Verification items for the finished model (mm, model axes). A direction names the side the tool comes from. Coordinates: 2 decimals unless noted, no trailing zeros. Write each loop counter-clockwise with the first axis right and the second up, starting at its lowest first coordinate (ties: lowest second). Pieces come first, ordered by that corner, then holes. Notation, with made-up numbers: (34.5, 45) -> (42.5, 45) arc R17 ccw to (42.5, 73) -> close; hole circle Ø10 at (41, 35). An arc over 180 degrees is marked (long way). Answer in a Markdown table with one row per item.
Autodesk Fusion 360 part; units mm, degrees
sketch "Sketch1" plane through (0, 0, 0) normal (0, 1, 0) x (1, 0, 0)
  line L0 (2.4744, -68.9852) -> (7.4744, -68.9852)
  line L1 (7.4744, -68.9852) -> (7.4744, -22.3387)
  line L2 (7.4744, -22.3387) -> (36.754, -10.3303)
  line L3 (36.754, -10.3303) -> (34.8567, -5.7042)
  line L4 (34.8567, -5.7042) -> (2.4744, -18.9852)
  line L5 (2.4744, -18.9852) -> (2.4744, -68.9852)
  line L6 (2.4744, -68.9852) -> (7.4744, -66.9345)
  line L7 (34.8567, -5.7042) -> (34.8567, -11.1084)
  dimension "d1" = 5
  dimension "d2" = 5
  dimension "d3" = 112.3
  dimension "d16" = 50
  dimension "d18" = 22.3
  dimension "d20" = 35
extrude "Extrude1" add sketch "Sketch1" along normal blind 220 contours L1 L2 L4 L5 L6 L7
sketch "Sketch2" plane through (2.4744, 0, 0) normal (-1, 0, 0) x (0, -1, 0)
  line L0 (0, 18.9852) -> (0, 68.9852)
  line L1 (-220, 68.9852) -> (-220, 18.9852)
  line L2 (-220, 18.9852) -> (0, 18.9852)
  line L3 (-215, 66.9852) -> (-5, 66.9852)
  line L4 (-5, 66.9852) -> (-5, 56.9852)
  line L5 (-5, 56.9852) -> (-215, 56.9852)
  line L6 (-215, 56.9852) -> (-215, 66.9852)
  line L7 (-215, 52.9852) -> (-5, 52.9852)
  line L8 (-5, 52.9852) -> (-5, 42.9852)
  line L9 (-5, 42.9852) -> (-215, 42.9852)
  line L10 (-215, 42.9852) -> (-215, 52.9852)
  line L11 (-5, 66.9852) -> (-15, 66.9852)
  line L12 (-15, 56.9852) -> (-5, 56.9852)
  line L13 (-5, 56.9852) -> (-5, 66.9852)
  line L14 (-5, 52.9852) -> (-15, 52.9852)
  line L15 (-15, 42.9852) -> (-5, 42.9852)
  line L16 (-5, 42.9852) -> (-5, 52.9852)
  line L17 (0, 68.9852) -> (-220, 68.9852)
  dimension "d6" = 210
  dimension "d7" = 210
  dimension "d8" = 5
  dimension "d9" = 5
  dimension "d12" = 10
  dimension "d13" = 10
  dimension "d22" = 4
  dimension "d30" = 2
extrude "Extrude2" cut sketch "Sketch2" against normal blind 3 contours L3 L4 L5 L6 L11 L12 L13 | L7 L8 L9 L10 L14 L15 L16
sketch "Sketch3" plane through (5.4744, 0, 0) normal (-1, 0, 0) x (0, -1, 0)
  line L0 (-215, 56.9852) -> (-5, 56.9852)
  line L1 (-5, 56.9852) -> (-5, 66.9852)
  line L2 (-5, 66.9852) -> (-215, 66.9852)
  line L3 (-215, 66.9852) -> (-215, 56.9852)
  line L4 (-5, 66.9852) -> (-15, 66.9852)
  line L5 (-15, 66.9852) -> (-15, 56.9852)
  line L6 (-15, 56.9852) -> (-5, 56.9852)
  line L7 (-5, 56.9852) -> (-5, 66.9852)
  dimension "d33" = 10
  dimension "d34" = 10
sketch "Sketch4" plane through (5.4744, 0, 0) normal (-1, 0, 0) x (0, -1, 0)
  line L0 (-215, 42.9852) -> (-5, 42.9852)
  line L1 (-5, 42.9852) -> (-5, 52.9852)
  line L2 (-215, 52.9852) -> (-215, 42.9852)
  line L3 (-5, 52.9852) -> (-15, 52.9852)
  line L4 (-15, 52.9852) -> (-15, 42.9852)
  line L5 (-15, 42.9852) -> (-5, 42.9852)
  line L6 (-5, 42.9852) -> (-5, 52.9852)
  line L7 (-5, 52.9852) -> (-215, 52.9852)
  dimension "d26" = 10
  dimension "d27" = 10
extrude "Extrude3" cut sketch "Sketch3" sketch "Sketch4" against normal blind 2 contours L0 L1 L2 L4 L5 L6 L7 of sketch 2 contours L0 L1 L3 L4 L5 L6 L7
equation "d4 = 200 mm + 10 mm + 5 mm + 5 mm"
equation "d6 = 200 mm + 10 mm"
equation "d7 = 200 mm + 10 mm"
1. Sectioned sample at D-D, the plane x = 31. Record the cut outline in (y, z), and give its area (3 significant figures).
Findings below:
| item | result |
|---|---|
| outline | (0, 7.29) -> (220, 7.29) -> (220, 12.69) -> (0, 12.69) -> close |
| area | 1,190 mm² |
2. Material ranges on probe 1 along Z at (x, y) = (5, 153); probe 2 along X at (y, z) = (45, 52); probe 3 along X at (y, z) = (125.5, 38), recorded low to high. Write a range as from..to.
Findings below:
| item | result |
|---|---|
| probe 1 | z = 17.95..42.99, 52.99..56.99, 66.99..67.95 |
| probe 2 | x = 5.47..7.47 |
| probe 3 | x = 2.47..7.47 |
3. Sectioned sample at C-C, the plane z = 33.5. Record the cut outline in (x, y), and give its area (3 significant figures).
Findings below:
| item | result |
|---|---|
| outline | (2.47, 0) -> (7.47, 0) -> (7.47, 220) -> (2.47, 220) -> close |
| area | 1,100 mm² |
4. Go/stop test with flat-tipped pins: pin 1 (8 mm diameter, centred on x = 31.5, y = 138, fed in from +Z); pin 2 (8 mm diameter, centred on x = 7.5, y = 70.5, fed in from -Z); pin 3 (1.5 mm diameter, centred on x = 4.5, y = 115.5, fed in from -Z). Record where each tip stops, or that it passes through.
Findings below:
| item | result |
|---|---|
| pin 1 | stops at z = 14.13 |
| pin 2 | stops at z = 15.28 |
| pin 3 | stops at z = 17.85 |
5. Sectioned sample at A-A, the plane z = 46.5. Record the cut outline in (x, y), and give its area (3 significant figures).
Findings below:
| item | result |
|---|---|
| outline | (2.47, 0) -> (7.47, 0) -> (7.47, 5) -> (2.47, 5) -> close; (2.47, 215) -> (5.47, 215) -> (5.47, 15) -> (7.47, 15) -> (7.47, 220) -> (2.47, 220) -> close |
| area | 450 mm² |
6. Access from +Z, -Z, +X, -X, +Y, -Y to the whole of each face (thin tool, end or side, straight path). Record for faces 1 (the face through (7, 220, 33)), 2 (the face through (5.474, 116, 48)), 3 (the face through (5, 5, 62)), 4 (the face through (7.474, 108, 45)).
Findings below:
| item | result |
|---|---|
| face 1 | +Z, -Z, +X, -X, +Y |
| face 2 | -X |
| face 3 | +X, -X |
| face 4 | +Z, +X, +Y, -Y |
7. Release check for a two-part mould opening along Z. For faces 5 (the face through (34.857, 108, 8)), 6 (the face through (18.892, 108.46, 12.252)), 7 (the face through (4, 109, 42.985)) record: released by +Z, released by -Z, zero draft, split by the parting line, or undercut.
Findings below:
| item | result |
|---|---|
| face 5 | zero draft |
| face 6 | released by -Z |
| face 7 | undercut |
8. Sectioned sample at B-B, the plane y = 79.5. Record the cut outline in (x, z).
Findings below:
| item | result |
|---|---|
| outline | (2.47, 18.99) -> (34.86, 5.7) -> (34.86, 11.11) -> (7.47, 22.34) -> (7.47, 66.93) -> (2.47, 68.99) -> (2.47, 66.99) -> (5.47, 66.99) -> (5.47, 56.99) -> (2.47, 56.99) -> (2.47, 52.99) -> (5.47, 52.99) -> (5.47, 42.99) -> (2.47, 42.99) -> close |
